from build123d import *

# Parameters (mm, degrees)
SKETCH_1_R                         = 1.5
SM_BASE_FLANGE_1_DEPTH             = 2
SM_EDGE_FLANGE_1_STRIP_W           = 9.4732
SM_EDGE_FLANGE_1_STRIP_H           = 2
SM_EDGE_FLANGE_1_STRIP_CUT_DEPTH   = 58
SM_EDGE_FLANGE_1_STRIP_2_W         = 9.4732
SM_EDGE_FLANGE_1_STRIP_2_H         = 2
SM_EDGE_FLANGE_1_STRIP_CUT_2_DEPTH = 58
SM_EDGE_FLANGE_1_DEPTH             = 58
SM_EDGE_FLANGE_1_BEND_DEPTH        = 58
SKETCH_12_R                        = 1.5
SKETCH_12_R_2                      = 8
CUT_EXTRUDE_1_DEPTH                = 10
SKETCH_21_R                        = 1.5
SKETCH_21_R_2                      = 8
CUT_EXTRUDE_2_DEPTH                = 10
CUT_EXTRUDE_3_DEPTH                = 102.712142835


# Sheet-metal steps are written as plain solids
with BuildPart() as part:
    # Sketch 1 → 基体-法兰1 (new body)
    with BuildSketch(Plane(origin=(0, 0, 0), x_dir=(1, 0, 0), z_dir=(0, 1, 0))):
        Polygon((-29, -36), (-29, 36), (-29, 38), (29, 38), (29, 36), (29, -36), (29, -36.4), (-29, -36.4), align=None)
        with Locations(Location((0, 13.5, 0), (0, 0, 270))):
            Circle(SKETCH_1_R, mode=Mode.SUBTRACT)
        with Locations(Location((11.691342951, 6.75, 0), (0, 0, 270))):
            Circle(SKETCH_1_R, mode=Mode.SUBTRACT)
        with Locations(Location((11.691342951, -6.75, 0), (0, 0, 270))):
            Circle(SKETCH_1_R, mode=Mode.SUBTRACT)
        with Locations(Location((0, -13.5, 0), (0, 0, 270))):
            Circle(SKETCH_1_R, mode=Mode.SUBTRACT)
        with Locations(Location((-11.691342951, -6.75, 0), (0, 0, 270))):
            Circle(SKETCH_1_R, mode=Mode.SUBTRACT)
        with Locations(Location((-11.691342951, 6.75, 0), (0, 0, 270))):
            Circle(SKETCH_1_R, mode=Mode.SUBTRACT)
    extrude(amount=-SM_BASE_FLANGE_1_DEPTH)

    # 边线-法兰1 strip (across the edge) → 边线-法兰1 strip cut (cut)
    with BuildSketch(Plane(origin=(29, 0, -38), x_dir=(0, 0, 1), z_dir=(-1, 0, 0))):
        with Locations((-2, -1)):
            Rectangle(SM_EDGE_FLANGE_1_STRIP_W, SM_EDGE_FLANGE_1_STRIP_H)
    extrude(amount=SM_EDGE_FLANGE_1_STRIP_CUT_DEPTH, mode=Mode.SUBTRACT)

    # 边线-法兰1 strip 2 (across the edge) → 边线-法兰1 strip cut 2 (cut)
    with BuildSketch(Plane(origin=(-29, 0, 36.4), x_dir=(0, 0, -1), z_dir=(1, 0, 0))):
        with Locations((-2, -1)):
            Rectangle(SM_EDGE_FLANGE_1_STRIP_2_W, SM_EDGE_FLANGE_1_STRIP_2_H)
    extrude(amount=SM_EDGE_FLANGE_1_STRIP_CUT_2_DEPTH, mode=Mode.SUBTRACT)

    # 边线-法兰1 section (across the edge) → 边线-法兰1 (add)
    with BuildSketch(Plane(origin=(29, 0, -38), x_dir=(0, 0, 1), z_dir=(-1, 0, 0))):
        with BuildLine():
            Line((0, 0.7366), (0, 63))
            Line((0, 63), (2, 63))
            Line((2, 63), (2, 0.7366))
            ThreePointArc((2, 0.7366), (2.215745145, 0.215745145), (2.7366, 0))
            Line((2.7366, 0), (2.7366, -2))
            ThreePointArc((2.7366, -2), (0.801531583, -1.198468417), (0, 0.7366))
        make_face()
    extrude(amount=SM_EDGE_FLANGE_1_DEPTH)

    # 边线-法兰1 section 2 (across the edge) → 边线-法兰1 bend (add)
    with BuildSketch(Plane(origin=(-29, 0, 36.4), x_dir=(0, 0, -1), z_dir=(1, 0, 0))):
        with BuildLine():
            Line((0, 0.7366), (0, 63))
            Line((0, 63), (2, 63))
            Line((2, 63), (2, 0.7366))
            ThreePointArc((2, 0.7366), (2.215745145, 0.215745145), (2.7366, 0))
            Line((2.7366, 0), (2.7366, -2))
            ThreePointArc((2.7366, -2), (0.801531583, -1.198468417), (0, 0.7366))
        make_face()
    extrude(amount=SM_EDGE_FLANGE_1_BEND_DEPTH)

    # 草图12 → 切除-拉伸1 (cut)
    with BuildSketch(Plane(origin=(0, 0, -38), x_dir=(-1, 0, 0), z_dir=(0, 0, -1))):
        with BuildLine():
            ThreePointArc((-29, 40.5), (-22.409902591, 56.409902563), (-6.50000004, 63))
            Line((-6.50000004, 63), (-29, 63))
            Line((-29, 63), (-29, 40.5))
        make_face()
        with Locations(Location((-6.5, 56.5, 0), (0, 0, 270))):
            Circle(SKETCH_12_R)
        with Locations(Location((7.356406461, 48.5, 0), (0, 0, 270))):
            Circle(SKETCH_12_R)
        with Locations(Location((-20.356406461, 48.5, 0), (0, 0, 270))):
            Circle(SKETCH_12_R)
        with Locations(Location((-20.356406461, 32.5, 0), (0, 0, 270))):
            Circle(SKETCH_12_R)
        with Locations(Location((-6.5, 24.5, 0), (0, 0, 270))):
            Circle(SKETCH_12_R)
        with Locations(Location((7.356406461, 32.5, 0), (0, 0, 270))):
            Circle(SKETCH_12_R)
        with Locations(Location((-6.5, 40.5, 0), (0, 0, 270))):
            Circle(SKETCH_12_R_2)
    extrude(amount=-CUT_EXTRUDE_1_DEPTH, mode=Mode.SUBTRACT)

    # 草图21 → 切除-拉伸2 (cut)
    with BuildSketch(Plane(origin=(0, 0, 34.4), x_dir=(-1, 0, 0), z_dir=(0, 0, -1))):
        with Locations((5.191342951, 47.25)):
            Circle(SKETCH_21_R)
        with Locations(Location((-6.5, 40.5, 0), (0, 0, 270))):
            Circle(SKETCH_21_R_2)
        with Locations((-6.5, 54)):
            Circle(SKETCH_21_R)
        with BuildLine():
            ThreePointArc((-29, 40.5), (-22.409902577, 56.409902577), (-6.5, 63))
            Line((-6.5, 63), (-29, 63))
            Line((-29, 63), (-29, 40.5))
        make_face()
        with Locations((-18.191342951, 47.25)):
            Circle(SKETCH_21_R)
        with Locations((-18.191342951, 33.75)):
            Circle(SKETCH_21_R)
        with Locations((-6.5, 27)):
            Circle(SKETCH_21_R)
        with Locations((5.191342951, 33.75)):
            Circle(SKETCH_21_R)
    extrude(amount=-CUT_EXTRUDE_2_DEPTH, mode=Mode.SUBTRACT)

    # 草图22 → 切除-拉伸3 (cut, through all)
    with BuildSketch(Plane(origin=(0, 0, -38), x_dir=(-1, 0, 0), z_dir=(0, 0, -1))):
        with BuildLine():
            Line((15.040771003, 46.999629574), (29, 0.7366))
            Line((29, 0.7366), (29, 63))
            Line((29, 63), (-6.5, 63))
            ThreePointArc((-6.5, 63), (6.91656317, 58.56227651), (15.040771003, 46.999629574))
        make_face()
    extrude(amount=-CUT_EXTRUDE_3_DEPTH, mode=Mode.SUBTRACT)


solid = part.part
Model file for the job. Use its own axes, mm. A direction names the side the tool comes from. Give positions to 0.01 mm unless a question says otherwise; leave off trailing zeros. Order: outer loops, then holes, each group sorted by start corner. A loop starts at its lowest first (then second) coordinate and runs counter-clockwise, first axis right, second up. Notation, with made-up numbers: (18.25, 44.25) -> (36.25, 44.25) arc R15 cw to (36.25, 62.25) -> close; hole circle Ø11 at (80.5, 10). An arc over 180 degrees is marked (long way). Use CSV: the item, a comma, the result in double quotes.
1. Drill centre lines: line 1 along X through (y, z) = (-0.85, 6.75); line 2 along Z through (x, y) = (16, 20); line 3 along Y through (x, z) = (15, 5). Where is each one in solid material? Low to high. Write a range as from..to.
Outcome:
line 1,"-29..-13.19, -10.19..10.19, 13.19..29"
line 2,"-38..-36, 34.4..36.4"
line 3,"-2..0"
2. Band-saw the part on D-D, the plane x = -24. Give the cut face in (y, z), then the cut area to 3 significant figures.
Outcome:
outline,"(-2, -35.26) arc R2.74 ccw to (0.74, -38) -> (17.31, -38) -> (17.31, -36) -> (0.74, -36) arc R0.74 cw to (0, -35.26) -> (0, 33.66) arc R0.74 cw to (0.74, 34.4) -> (17.31, 34.4) -> (17.31, 36.4) -> (0.74, 36.4) arc R2.74 ccw to (-2, 33.66) -> close"
area,"215 mm²"
3. 3-axis set-ups, long thin cutter, end or side, ignore diameter. For faces 5 (the cylindrical face through (-4.866, 45.786, 35.386)), 6 (the cylindrical face through (11.368, 46.849, -37.014)), 7 (the cylindrical face through (-10.68, -0.99, 5.64)), 8 (the flat face through (0, 25, -36)), 9 (the cylindrical face through (-7.4, 50, -37)): which of +Z, -Z, +X, -X, +Y, -Y reach the whole face in a straight line?
Outcome:
face 5,"+Z"
face 6,"+Z, -Z"
face 7,"+Y, -Y"
face 8,"+X, -X, +Y"
face 9,"-Z"
4. Mould opens along Y. For faces 1 (the cylindrical face through (6.825, 52.536, 35.386)), 2 (the flat face through (0, 25, -38)), 3 (the cylindrical face through (0.406, -1.22, -37.177)), 4 (the flat face through (-21.923, 24.192, 35.386)) say: +Y half, -Y half, draft (parallel to the pull), parting line (faces both ways), or undercut.
Outcome:
face 1,"undercut"
face 2,"draft"
face 3,"-Y half"
face 4,"+Y half"
5. Band-saw the part on A-A, the plane z = 13.5. Give the cut face in (x, y).
Outcome:
outline,"(-29, -2) -> (-1.5, -2) -> (-1.5, 0) -> (-29, 0) -> close; (1.5, -2) -> (29, -2) -> (29, 0) -> (1.5, 0) -> close"
6. Band-saw the part on B-B, the plane y = 54. Give the cut face in (x, z), then the cut area to 3 significant figures.
Outcome:
outline,"(-11.5, -38) -> (24.5, -38) -> (24.5, -36) -> (-11.5, -36) -> close; (-11.5, 34.4) -> (5, 34.4) -> (5, 36.4) -> (-11.5, 36.4) -> close; (8, 34.4) -> (24.5, 34.4) -> (24.5, 36.4) -> (8, 36.4) -> close"
area,"138 mm²"
7. Drop flat-ended pins along their axis: pin 1 (1.8 mm diameter, centred on x = 11.69, z = -6.75, fed in from +Y); pin 2 (2.5 mm diameter, centred on x = 6.5, y = 56.5, fed in from -Z); pin 3 (3.5 mm diameter, centred on x = -7.36, y = 32.5, fed in from -Z); pin 4 (17.5 mm diameter, centred on x = 5, z = -3, fed in from +Y). Give the stop position or say it passes through.
Outcome:
pin 1,"through"
pin 2,"z = 34.4"
pin 3,"z = -38"
pin 4,"y = 0"
8. Band-saw the part on C-C, the plane y = 18. Give the cut face in (x, z), then the cut area to 3 significant figures.
Outcome:
outline,"(-23.79, -38) -> (29, -38) -> (29, -36) -> (-23.79, -36) -> close; (-23.79, 34.4) -> (29, 34.4) -> (29, 36.4) -> (-23.79, 36.4) -> close"
area,"211 mm²"
